```python
from build123d import *

# Parameters (mm, degrees)
BOSS_EXTRU_1_DEPTH                              = 7
CHAMBRAGE_POUR_VIS_T_TE_CYLINDRIQUE_D           = 3.2
CHAMBRAGE_POUR_VIS_T_TE_CYLINDRIQUE_CBORE_D     = 6
CHAMBRAGE_POUR_VIS_T_TE_CYLINDRIQUE_CBORE_DEPTH = 3
CONG_1_R                                        = 2
ESQUISSE5_R                                     = 1.6
ENL_V_MAT_EXTRU_1_DEPTH                         = 10
ENL_V_START                                     = -3
ENL_V_MAT_EXTRU_2_DEPTH                         = 7


with BuildPart() as part:
    # Esquisse1 → Boss.-Extru.1 (new, symmetric)
    with BuildSketch(Plane(origin=(0, 0, 0), x_dir=(1, 0, 0), z_dir=(0, 1, 0))):
        with BuildLine():
            Line((-10, 0), (-10, -7))
            Line((-10, -7), (3, -7))
            ThreePointArc((3, -7), (7.186709482, -9.064656631), (8.097414494, -13.643079905))
            Line((8.097414494, -13.643079905), (3.446641772, -31))
            Line((3.446641772, -31), (10.693575035, -31))
            Line((10.693575035, -31), (19, 0))
            Line((19, 0), (-10, 0))
        make_face()
    extrude(amount=BOSS_EXTRU_1_DEPTH, both=True)

    # Chambrage pour vis à tête cylindrique à 6 pans creux (ou vis CHC) M31 (through all)
    with Locations(Plane.XY.offset(7)):
        with Locations((0, 0)):
            CounterBoreHole(CHAMBRAGE_POUR_VIS_T_TE_CYLINDRIQUE_D / 2, CHAMBRAGE_POUR_VIS_T_TE_CYLINDRIQUE_CBORE_D / 2, CHAMBRAGE_POUR_VIS_T_TE_CYLINDRIQUE_CBORE_DEPTH)

    # Congé1
    cong_1_edges = [part.edges().sort_by_distance(p)[0] for p in [
        (10.693575035, 0, 31),
        (3.446641772, 0, 31),
        (-10, 0, 7),
    ]]
    fillet(cong_1_edges, radius=CONG_1_R)

    # Esquisse5 → Enlèv. mat.-Extru.1 (cut)
    with BuildSketch(Plane(origin=(17.727241336, 0, 4.75), x_dir=(0.25881904510252474, 0, -0.9659258262890673), z_dir=(0.9659258262890673, 0, 0.25881904510252474))):
        with Locations((-10.082438143, 0)):
            Circle(ESQUISSE5_R)
    extrude(amount=-ENL_V_MAT_EXTRU_1_DEPTH, mode=Mode.SUBTRACT)

    # Esquisse6 → Enlèv. mat.-Extru.2 (cut)
    with BuildSketch(Plane(origin=(17.727241336, 0, 4.75), x_dir=(0.25881904510252474, 0, -0.9659258262890673), z_dir=(0.9659258262890673, 0, 0.25881904510252474)).offset(ENL_V_START)):
        Polygon((-7.332438143, 1.58771324), (-10.082438143, 3.175426481), (-12.832438143, 1.58771324), (-12.832438143, -1.58771324), (-10.082438143, -3.175426481), (-7.332438143, -1.58771324), align=None)
    extrude(amount=-ENL_V_MAT_EXTRU_2_DEPTH, mode=Mode.SUBTRACT)


solid = part.part
```
The listing builds one solid part. Answer for the finished solid, in the listing's coordinates (mm). A direction names the side the tool comes from. Coordinates: 2 decimals unless noted, no trailing zeros. Loops run counter-clockwise (first coordinate to the right, second up) from the corner with the lowest first, then second, coordinate; pieces in that order, holes last. Notation, with made-up numbers: (11, 45) -> (16, 45) arc R5 ccw to (16, 50) -> close; hole circle Ø7 at (4, -18.75). An arc over 180 degrees is marked (long way). Use one line per item in the form item = value. Start each with the question number.
Item 1: The part is cut by section A-A on x = 0. Determine the outline of the cut face in (y, z), then the cut area to 3 significant figures.
Item 2: Consider L1, parallel to Y at x = 0, z = 5.55; L2, parallel to Z at x = -1.5, y = -3.5; L3, parallel to Y at x = 10.25, z = 12. Determine where each line is inside the solid, lowest interval first. Write a range as [from, to].
Item 3: The mould has two halves that part along Y. Classify faces 6 (the face through (8, 0, 31)), 7 (the face through (1.27, -0.97, 1.97)): released by +Y, released by -Y, zero draft, split by the parting line, or undercut.
Item 4: A tool of negligible diameter and unlimited length cuts with its end or side. For faces 1 (the face through (14.99, 3.21, 14.97)), 2 (the face through (11.9, -1.4, 14.9)), 3 (the face through (6.137, 0.098, 20.959)), 4 (the face through (-4, 0, 7)), 5 (the face through (1.3, -1.3, 4)), from which of +Z, -Z, +X, -X, +Y, -Y can it reach the whole face along a straight path? Write none if from no direction.
Item 5: The part is cut by section D-D on x = 3.5. Determine the outline of the cut face in (y, z).
Item 6: The part is cut by section C-C on z = 11.5. Determine the outline of the cut face in (x, y), then the cut area to 3 significant figures.
Item 7: Flat-ended cylindrical pins translate along their axes: pin 1 Ø6 at (x, y) = (-2, 3) entering from +Z; pin 2 Ø1.5 at (x, y) = (3, -0.5) entering from +Z; pin 3 Ø1.5 at (y, z) = (2.5, 7) entering from -X. Find the tip coordinate at first contact, or state that the pin passes through.
Item 8: The part is cut by section B-B on y = 5. Determine the outline of the cut face in (x, z), then the cut area to 3 significant figures.
Answer key:
q1.outline = (-7, 0) -> (-1.6, 0) -> (-1.6, 4) -> (-3, 4) -> (-3, 7) -> (-7, 7) -> close; (1.6, 0) -> (7, 0) -> (7, 7) -> (3, 7) -> (3, 4) -> (1.6, 4) -> close
q1.area = 67.2 mm2
q2.L1 = [-7, -3], [3, 7]
q2.L2 = [0, 7]
q2.L3 = [-7, -2.51], [2.51, 7]
q3.face_6 = zero draft
q3.face_7 = undercut
q4.face_1 = +Z, +X, +Y, -Y
q4.face_2 = none
q4.face_3 = -X, +Y, -Y
q4.face_4 = +Z, -X, +Y, -Y
q4.face_5 = +Z
q5.outline = (-7, 0) -> (7, 0) -> (7, 7.02) -> (-7, 7.02) -> close
q6.outline = (8.22, -7) -> (15.92, -7) -> (15.92, 7) -> (8.22, 7) -> (8.22, 2.54) -> (12.81, 1.85) -> (12.81, -1.85) -> (8.22, -2.54) -> close
q6.area = 87.6 mm2
q7.pin_1 = 7
q7.pin_2 = 7.05
q7.pin_3 = -9.56
q8.outline = (-10, 0) -> (19, 0) -> (11.09, 29.52) arc R2 ccw to (9.16, 31) -> (6.05, 31) arc R2 ccw to (4.12, 28.48) -> (8.1, 13.64) arc R5.28 cw to (3, 7) -> (-8, 7) arc R2 ccw to (-10, 5) -> close
q8.area = 378 mm2
